The listing builds one solid part. Answer for the finished solid, in the listing's coordinates (mm). Face numbers are marked on the shaded views. A direction names the side the tool comes from. Give positions to 0.01 mm unless a question says otherwise; leave off trailing zeros. Write each loop counter-clockwise with the first axis right and the second up, starting at its lowest first coordinate (ties: lowest second). Pieces come first, ordered by that corner, then holes.
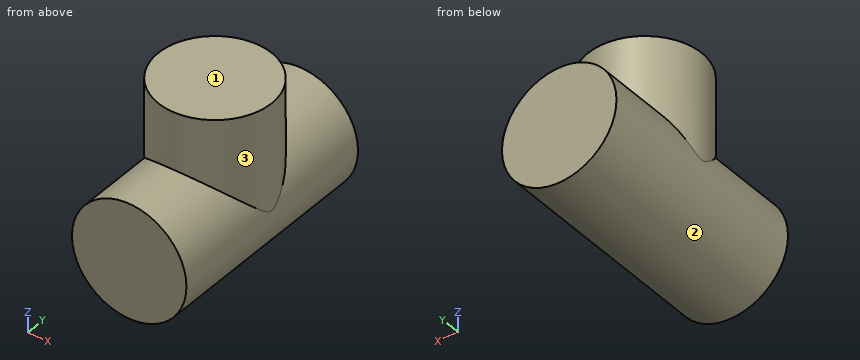
```python
from build123d import *

# Parameters (mm, degrees)
F0_R      = 38.093898
F1_DEPTH  = 76.2
F1_FACE_R = 38.093898
F2_DEPTH  = 76.2
F3_R      = 37.724218
F4_DEPTH  = 76.2


with BuildPart() as f1:
    # F0 (on Front) → F1 (new body)
    with BuildSketch(Plane.XZ):
        Circle(F0_R)
    extrude(amount=F1_DEPTH)

    # F0 (on Front) + F1_face (on face) → F2 (join)
    with BuildSketch(Plane.XZ):
        Circle(F0_R)
    with BuildSketch(Plane(origin=(0, 0, 0), x_dir=(1, 0, 0), z_dir=(0, 1, 0))):
        Circle(F1_FACE_R)
    extrude(amount=-F2_DEPTH)

    # F3 (on Top) → F4 (join)
    with BuildSketch(Plane.XY):
        Circle(F3_R)
    extrude(amount=F4_DEPTH)


solid = f1.part
```
Item 1: Consider probe 1 along Z at (x, y) = (1, 29.5); probe 2 along X at (y, z) = (-1, 50); probe 3 along Z at (x, y) = (-34, -60.5). Determine where each line is inside the solid, lowest interval first.
Conclusion:
probe 1: z = -38.08 to 76.2
probe 2: x = -37.71 to 37.71
probe 3: z = -17.18 to 17.18
Item 2: A cutting plane is placed at B-B, the plane x = -32. Give the vertices of the cut face in (y, z), plus the area to 3 significant figures.
Conclusion:
outline: (-76.2, -20.67) - (76.2, -20.67) - (76.2, 20.67) - (19.98, 20.67) - (19.98, 76.2) - (-19.98, 76.2) - (-19.98, 20.67) - (-76.2, 20.67) - close
area: 8,520 mm2
Item 3: A cutting plane is placed at D-D, the plane z = 44. Give the vertices of the cut face in (x, y), plus the area to 3 significant figures.
Conclusion:
outline: circle Ø75.45 at (0, 0)
area: 4,470 mm2
Item 4: A cutting plane is placed at A-A, the plane z = 30. Give the vertices of the cut face in (x, y).
Conclusion:
outline: (-23.48, -76.2) - (23.48, -76.2) - (23.48, -29.53) arc R37.72 ccw to (23.48, 29.53) - (23.48, 76.2) - (-23.48, 76.2) - (-23.48, 29.53) arc R37.72 ccw to (-23.48, -29.53) - close
Item 5: A cutting plane is placed at C-C, the plane y = 0. Give the vertices of the cut face in (x, z), plus the area to 3 significant figures.
Conclusion:
outline: (-37.72, 5.29) arc R38.09 ccw (long way) to (37.72, 5.29) - (37.72, 76.2) - (-37.72, 76.2) - close
area: 8,030 mm2
Item 6: Which of the six approach directions +Z, -Z, +X, -X, +Y, -Y give full straight-line access (tool end or side, diameter ignored) to the marked faces 1, 2 and 3?
Conclusion:
face 1: +Z, +X, -X, +Y, -Y
face 2: none
face 3: +Z
Item 7: Each of these flat-tipped pins is pushed along its axis until it touches: P1, Ø1, axis at y = -16.5, z = 48.5, coming from the +X side; P2, Ø1.5, axis at y = -4, z = 52.5, coming from the -X side; P3, Ø4, axis at x = 3.5, z = 52, coming from the -Y side. Where does it stop, or does it pass through?
Conclusion:
P1: stops at x = 34.16
P2: stops at x = -37.58
P3: stops at y = -37.69
